Print and shaded views of the part. All mm, measured from the part's lowest x, y and z. Coordinates: 2 decimals unless noted, no trailing zeros. Loops run counter-clockwise (first coordinate to the right, second up) from the corner with the lowest first, then second, coordinate; pieces in that order, holes last. Notation, with made-up numbers: M 32.5,48.25 L 71.5,48.25 A12 cw 71.5,54.25 Z; hole C 18,23.25 d1. An arc over 180 degrees is marked long. Answer as a JSON object with one key per item and string values. Group by question number.
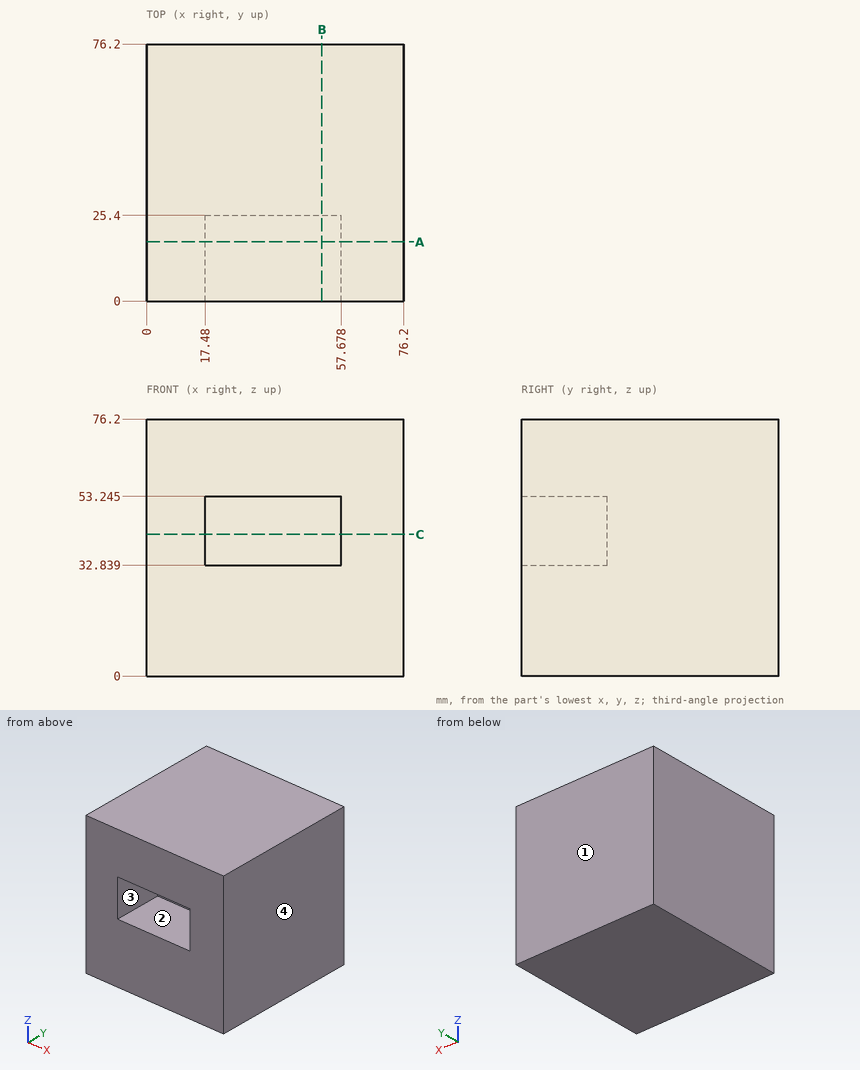
Item 1: Slice it at B-B, the plane x = 52. Write the cut outline in (y, z) (1 decimal), then the cut area to 3 significant figures.
Item 2: Drill centre lines: L1, parallel to X at y = 13, z = 46; L2, parallel to Z at x = 33.5, y = 12.5 (1 decimal); L3, parallel to Y at x = 56, z = 43. Where is each one in solid material? Low to high. Write a range as from..to.
Item 3: Pull direction X, two halves, no side cores. Call the marked faces 1, 2, 3 and 4: released by +X, released by -X, zero draft, split by the parting line, or undercut.
Item 4: Slice it at C-C, the plane z = 42. Write the cut outline in (x, y).
Item 5: Slice it at A-A, the plane y = 17.5. Write the cut outline in (x, z) (1 decimal), then the cut area to 3 significant figures.
Computed:
{
 "1": {"outline": "M 0,0 L 76.2,0 L 76.2,76.2 L 0,76.2 L 0,53.2 L 25.4,53.2 L 25.4,32.8 L 0,32.8 Z", "area": "5,290 mm2"},
 "2": {"L1": "0..17.48, 57.68..76.2", "L2": "0..32.8, 53.2..76.2", "L3": "25.4..76.2"},
 "3": {"face 1": "zero draft", "face 2": "undercut", "face 3": "undercut", "face 4": "released by +X"},
 "4": {"outline": "M 0,0 L 17.48,0 L 17.48,25.4 L 57.68,25.4 L 57.68,0 L 76.2,0 L 76.2,76.2 L 0,76.2 Z"},
 "5": {"outline": "M 0,0 L 76.2,0 L 76.2,76.2 L 0,76.2 Z; hole M 17.5,32.8 L 57.7,32.8 L 57.7,53.2 L 17.5,53.2 Z", "area": "4,990 mm2"}
}
